Geometry: final body of the model. Coordinates: model frame, mm. Give positions to 0.01 mm unless a question says otherwise; leave off trailing zeros. Write each loop counter-clockwise with the first axis right and the second up, starting at its lowest first coordinate (ties: lowest second). Pieces come first, ordered by that corner, then holes. Notation, with made-up numbers: (-3.5, 34.25) -> (28.5, 34.25) arc R25 cw to (28.5, 66.25) -> close; hole circle Ø10 at (-34, 62.25). An arc over 180 degrees is marked (long way). Answer as a JSON object with one key per item and string values. Group by question number.
(1) Section query A-A on x = 23.5. Output: boundary loops of the cut face in (y, z).
(2) Section query C-C on z = -20.5. Output: boundary loops of the cut face in (x, y).
(3) Material intervals for probe 1 along Y at (x, z) = (22, -7); probe 2 along Z at (x, y) = (49, 14), sorted ascending.
(4) Section query D-D on x = 49. Output: boundary loops of the cut face in (y, z), plus the area to 3 significant figures.
(5) Draft query along Z for faces 1 (the face through (16, 0, 12.5)), 2 (the face through (16, 0, -12.5)), 3 (the face through (0, 0, 0)). Return one class per face: +Z half, -Z half, draft (parallel to the pull), parting line (faces both ways), or undercut.
(6) Section query B-B on y = 1. Output: boundary loops of the cut face in (x, z).
(7) Contact query for flat-ended pins moving along their axis: pin 1 Ø7.5 at (x, y) = (16.5, -5) entering from +Z; pin 2 Ø1 at (x, y) = (42, -7) entering from +Z; pin 3 Ø20 at (x, z) = (13.5, -4) entering from +Y; pin 4 Ø8 at (x, z) = (53, -1.5) entering from +Y. Output: stop coordinate, or through.
from build123d import *

# Parameters (mm, degrees)
F2_W     = 25
F2_H     = 25
F3_REACH = 110.3563390593


with BuildPart() as f1:
    # F0 (on Front) → F1 (revolve)
    with BuildSketch(Plane.XZ):
        with BuildLine():
            Line((0, 12.5), (0, 0))
            Line((0, 0), (25, 0))
            Line((25, 0), (50, 0))
            Line((50, 0), (75, 0))
            ThreePointArc((75, 0), (56.4704761276, 24.1481456572), (28.3493649054, 12.5))
            Line((28.3493649054, 12.5), (0, 12.5))
        make_face()
    revolve(axis=Axis((12.5, 0, 0), (1, 0, 0)))

    f3_end = f1.faces().sort_by_distance((56.4704761276, 0, -24.1481456572))[0]
    # F2 (on face) → F3 (join, up to a face of the model that its end follows)
    with BuildSketch(Plane(origin=(0, 0, 0), x_dir=(0, -1, 0), z_dir=(-1, 0, 0))):
        Rectangle(F2_W, F2_H)
    f3_long = extrude(amount=-F3_REACH, mode=Mode.PRIVATE)
    add(split(f3_long, bisect_by=f3_end, keep=Keep.ALL, mode=Mode.PRIVATE).solids().sort_by_distance((0, 0, 0))[0])


solid = f1.part
Answer list:
{
 "1": {"outline": "(-12.5, -12.5) -> (12.5, -12.5) -> (12.5, 12.5) -> (-12.5, 12.5) -> close"},
 "2": {"outline": "circle Ø28.62 at (50, 0)"},
 "3": {"probe 1": "-12.5 to 12.5", "probe 2": "-20.69 to 20.69"},
 "4": {"outline": "circle Ø49.96 at (0, 0)", "area": "1,960 mm2"},
 "5": {"face 1": "+Z half", "face 2": "-Z half", "face 3": "draft"},
 "6": {"outline": "(0, -12.5) -> (28.37, -12.5) arc R24.98 ccw (long way) to (28.37, 12.5) -> (0, 12.5) -> close"},
 "7": {"pin 1": "z = 12.5", "pin 2": "z = 22.86", "pin 3": "y = 12.5", "pin 4": "y = 25"}
}
